```python
from build123d import *

# Parameters (mm, degrees)
SKETCH_1_R      = 8
EXTRUDE_1_DEPTH = 120


with BuildPart() as part:
    # 草图1 → 凸台-拉伸1 (new, symmetric)
    with BuildSketch(Plane(origin=(0, 0, 0), x_dir=(1, 0, 0), z_dir=(0, 1, 0))):
        with Locations(Location((0, 0, 0), (0, 0, 270))):
            Circle(SKETCH_1_R)
    extrude(amount=EXTRUDE_1_DEPTH, both=True)

    # 草图3 → M6 螺纹孔1 (revolve, cut)
    with BuildSketch(Plane(origin=(0, 120, 0), x_dir=(0, 0, 1), z_dir=(1, 0, 0))):
        Polygon((0, 0), (0, 18.502151548), (2.5, 17), (2.5, 0), align=None)
    hole_wizard_m6_1 = revolve(axis=Axis((0, 126.35, 0), (0, -1, 0)), mode=Mode.SUBTRACT)

    # 镜向1: M6 螺纹孔1 across plane
    add(hole_wizard_m6_1.mirror(Plane.ZX), mode=Mode.SUBTRACT)


solid = part.part
```
CAD build for the part. Positions are in the model's coordinates, mm. A direction names the side the tool comes from. Coordinates: 2 decimals unless noted, no trailing zeros. Write each loop counter-clockwise with the first axis right and the second up, starting at its lowest first coordinate (ties: lowest second). Pieces come first, ordered by that corner, then holes. Notation, with made-up numbers: (-9.5, 83) -> (31.5, 83) arc R26 ccw to (31.5, 105) -> close; hole circle Ø2 at (-22, 48). An arc over 180 degrees is marked (long way). Use CSV: the item, a comma, the result in double quotes. Start each with the question number.
Item 1: Drop flat-ended pins along their axis: P1, Ø3, axis at x = 6, y = 17.5, coming from the +Z side; P2, Ø1, axis at y = 79, z = 4, coming from the -X side; P3, Ø1, axis at x = 6, y = -52, coming from the -Z side. Give the stop position or say it passes through.
Item 2: Two-plate mould, pull along Z, no slides. Class faces 4 (the flat face through (2, 120, 2)), 5 (the conical face through (0.424, -101.759, -0.094)), 6 (the cylindrical face through (-7.81, 1.68, -1.73)): +Z half, -Z half, draft (parallel to the pull), parting line (faces both ways), or undercut.
Item 3: Tool access for faces 1 (the flat face through (2, -120, 2)), 2 (the cylindrical face through (2.44, -111.62, -0.54)), 3 (the cylindrical face through (2.44, 111.62, -0.54)): list every direction of +Z, -Z, +X, -X, +Y, -Y with a clear straight run to the whole face (end or side of a thin tool).
Item 4: Band-saw the part on C-C, the plane z = 5.25. Write the cut outline in (x, y), plus the area to 3 significant figures.
Item 5: Band-saw the part on B-B, the plane x = -5. Write the cut outline in (y, z) (3 decimals), plus the area to 3 significant figures.
Item 6: Band-saw the part on A-A, the plane y = -46. Write the cut outline in (x, z).
Item 7: Wall check: probe 1 along X at (y, z) = (111, 0); probe 2 along Z at (x, y) = (-0.25, -16.5); probe 3 along X at (y, z) = (80, 0.5). Give the ranges that are in metal, low to high.
Response values:
1,P1,"stops at z = 6.61"
1,P2,"stops at x = -7.19"
1,P3,"stops at z = -5.81"
2,face 4,"draft"
2,face 5,"undercut"
2,face 6,"parting line"
3,face 1,"+Z, -Z, +X, -X, -Y"
3,face 2,"-Y"
3,face 3,"+Y"
4,outline,"(-6.04, -120) -> (6.04, -120) -> (6.04, 120) -> (-6.04, 120) -> close"
4,area,"2,900 mm2"
5,outline,"(-120, -6.245) -> (120, -6.245) -> (120, 6.245) -> (-120, 6.245) -> close"
5,area,"3,000 mm2"
6,outline,"circle Ø16 at (0, 0)"
7,probe 1,"x = -8 to -2.5, 2.5 to 8"
7,probe 2,"z = -8 to 8"
7,probe 3,"x = -7.98 to 7.98"
